```python
from build123d import *

# Parameters (mm, degrees)
BASPROSKE_W         = 10
BASPROSKE_H         = 12
TOOTHCUT_DEPTH      = 20.697715604
TEETHCUTS_COUNT     = 10
TEETHCUTS_ANGLE     = 324
BORSKE_R            = 2.5
BORE_DEPTH          = 50.0000508
BOSS_EXTRUDE1_DEPTH = 10


with BuildPart() as part:
    # BasProSke → Base-Revolve (revolve)
    with BuildSketch(Plane(origin=(0, 0, 0), x_dir=(1, 0, 0), z_dir=(0, 1, 0)), mode=Mode.PRIVATE) as base_revolve_sk:
        with Locations((5, 6)):
            Rectangle(BASPROSKE_W, BASPROSKE_H)
    revolve(base_revolve_sk.sketch.rotate(Axis((-10, 0, 0), (1, 0, 0)), 180), axis=Axis((-10, 0, 0), (1, 0, 0)))

    # TooCutSke → ToothCut (cut, through all)
    with BuildSketch(Plane(origin=(0, 0, 0), x_dir=(0, 0, -1), z_dir=(1, 0, 0))):
        with BuildLine():
            ThreePointArc((1.173662691, 7.406586048), (0, 7.499), (-1.173662691, 7.406586048))
            ThreePointArc((-1.173662691, 7.406586048), (-1.668191438, 9.834565786), (-3.497907776, 11.50542856))
            ThreePointArc((-3.497907776, 11.50542856), (0, 12.0254), (3.497907776, 11.50542856))
            ThreePointArc((3.497907776, 11.50542856), (1.668191438, 9.834565786), (1.173662691, 7.406586048))
        make_face()
    toothcut = extrude(amount=TOOTHCUT_DEPTH, mode=Mode.SUBTRACT)

    # TeethCuts: ToothCut ×10 about axis
    teethcuts_axis = Axis((-10, 0, 0), (1, 0, 0))
    for i in range(1, TEETHCUTS_COUNT):
        add(toothcut.rotate(teethcuts_axis, i * TEETHCUTS_ANGLE / (TEETHCUTS_COUNT - 1)), mode=Mode.SUBTRACT)

    # BorSke → Bore (cut, symmetric)
    with BuildSketch(Plane(origin=(0, 0, 0), x_dir=(0, 0, -1), z_dir=(1, 0, 0))):
        with Locations(Location((0, 0, 0), (0, 0, 180))):
            Circle(BORSKE_R)
    extrude(amount=BORE_DEPTH, both=True, mode=Mode.SUBTRACT)

    # Sketch1 → Boss-Extrude1 (add)
    with BuildSketch(Plane(origin=(10, 0, 0), x_dir=(0, 0, -1), z_dir=(1, 0, 0))):
        with BuildLine():
            Line((-1.660598254, 1.8688), (1.660598254, 1.8688))
            ThreePointArc((1.660598254, 1.8688), (0, 2.5), (-1.660598254, 1.8688))
        make_face()
    extrude(amount=-BOSS_EXTRUDE1_DEPTH)


solid = part.part
```
Geometry: final body of the model. Coordinates: model frame, mm. Give positions to 0.01 mm unless a question says otherwise; leave off trailing zeros. Order: outer loops, then holes, each group sorted by start corner. A loop starts at its lowest first (then second) coordinate and runs counter-clockwise, first axis right, second up. Notation, with made-up numbers: (36, -18) -> (73, -18) arc R28 ccw to (73, 3) -> close; hole circle Ø7 at (-17.5, 40.25). An arc over 180 degrees is marked (long way). Write each question's results on one line, items separated by ' | '. Start each with the question number.
1) First-contact query: pin 1 (5 mm diameter, centred on x = 4, y = -3, fed in from +Z); pin 2 (2.5 mm diameter, centred on x = 6.5, z = -0.5, fed in from -Y); pin 3 (4 mm diameter, centred on x = 5, z = -7.5, fed in from -Y). Flat tips, straight axial feed; report the tip coordinate or a pass-through.
2) Section A-A (z = 0). Return loops of the section in (x, y).
3) Section C-C (z = 9.25). Return loops of the section in (x, y), then the cut area to 3 significant figures.
4) Line query: line 1 (Z direction, x = 6.75, y = 0); line 2 (Y direction, x = 6.75, z = 0); line 3 (Y direction, x = 7.25, z = -8.5). Output: solid intervals per line, ascending. Write a range as from..to.
5) Section D-D (y = -3). Return loops of the section in (x, z), then the cut area to 3 significant figures.
6) Section B-B (y = 6). Return loops of the section in (x, z).
Calculated:
1) pin 1: z = 11.75 | pin 2: y = -9.97 | pin 3: y = -7.33
2) outline: (0, -7.5) -> (10, -7.5) -> (10, -2.5) -> (0, -2.5) -> close; (0, 1.87) -> (10, 1.87) -> (10, 7.5) -> (0, 7.5) -> close
3) outline: (0, -7.31) -> (10, -7.31) -> (10, -5.16) -> (0, -5.16) -> close; (0, -1.53) -> (10, -1.53) -> (10, 1.53) -> (0, 1.53) -> close; (0, 5.16) -> (10, 5.16) -> (10, 7.31) -> (0, 7.31) -> close | area: 73.5 mm2
4) line 1: -12..-2.5, 2.5..12 | line 2: -7.5..-2.5, 1.87..7.5 | line 3: -7.32..-4.3, -1.49..1.49, 4.3..7.32
5) outline: (0, -6.87) -> (10, -6.87) -> (10, 6.87) -> (0, 6.87) -> close | area: 137 mm2
6) outline: (0, -9.66) -> (10, -9.66) -> (10, -5.8) -> (0, -5.8) -> close; (0, -4.5) -> (10, -4.5) -> (10, 4.5) -> (0, 4.5) -> close; (0, 5.8) -> (10, 5.8) -> (10, 9.66) -> (0, 9.66) -> close
